The listing builds one solid part. Answer for the finished solid, in the listing's coordinates (mm). Give positions to 0.01 mm unless a question says otherwise; leave off trailing zeros. Write each loop counter-clockwise with the first axis right and the second up, starting at its lowest first coordinate (ties: lowest second). Pieces come first, ordered by that corner, then holes. Notation, with made-up numbers: (72, -26.5) - (101, -26.5) arc R33 ccw to (101, 12.5) - close; hole circle Ø4 at (63, -7). An arc over 180 degrees is marked (long way). Return JSON: item names as keys, results as strings.
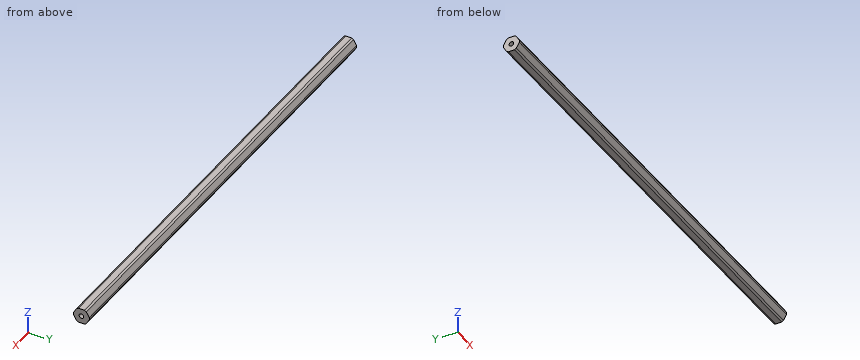
from build123d import *

# Parameters (mm, degrees)
BOSS_EXTRUDE1_DEPTH                  = 200.025
F_10_32_TAPPED_HOLE1_D               = 4.0386
F_10_32_TAPPED_HOLE1_DEPTH           = 16.34744
F_10_32_TAPPED_HOLE1_TIP             = 1.213317848
F_10_32_TAPPED_HOLE1_ON_FACE_2_D     = 4.0386
F_10_32_TAPPED_HOLE1_ON_FACE_2_DEPTH = 16.34744
F_10_32_TAPPED_HOLE1_ON_FACE_2_TIP   = 1.213317848


with BuildPart() as part:
    # Sketch1 → Boss-Extrude1 (new, symmetric)
    with BuildSketch(Plane(origin=(0, 0, 0), x_dir=(0, 0, -1), z_dir=(1, 0, 0))):
        with BuildLine():
            ThreePointArc((0.93173274, 6.79441227), (0, 6.858), (-0.93173274, 6.79441227))
            Line((-0.93173274, 6.79441227), (-5.41826726, 4.204110358))
            ThreePointArc((-5.41826726, 4.204110358), (-5.939202219, 3.429), (-6.35, 2.590301913))
            Line((-6.35, 2.590301913), (-6.35, -2.590301913))
            ThreePointArc((-6.35, -2.590301913), (-5.939202219, -3.429), (-5.41826726, -4.204110358))
            Line((-5.41826726, -4.204110358), (-0.93173274, -6.79441227))
            ThreePointArc((-0.93173274, -6.79441227), (0, -6.858), (0.93173274, -6.79441227))
            Line((0.93173274, -6.79441227), (5.41826726, -4.204110358))
            ThreePointArc((5.41826726, -4.204110358), (5.939202219, -3.429), (6.35, -2.590301913))
            Line((6.35, -2.590301913), (6.35, 2.590301913))
            ThreePointArc((6.35, 2.590301913), (5.939202219, 3.429), (5.41826726, 4.204110358))
            Line((5.41826726, 4.204110358), (0.93173274, 6.79441227))
        make_face()
    extrude(amount=BOSS_EXTRUDE1_DEPTH, both=True)

    # #10-32 Tapped Hole1
    with Locations(Plane(origin=(-200.025, 0, 0), x_dir=(0, 0, -1), z_dir=(-1, 0, 0))):
        with Locations((0, 0)):
            Hole(F_10_32_TAPPED_HOLE1_D / 2, depth=F_10_32_TAPPED_HOLE1_DEPTH)
            with Locations((0, 0, -(F_10_32_TAPPED_HOLE1_DEPTH + F_10_32_TAPPED_HOLE1_TIP / 2))):  # 118° drill point
                Cone(0, F_10_32_TAPPED_HOLE1_D / 2, F_10_32_TAPPED_HOLE1_TIP, mode=Mode.SUBTRACT)

    # #10-32 Tapped Hole1 on face 2
    with Locations(Plane(origin=(200.025, 0, 0), x_dir=(0, 0, 1), z_dir=(1, 0, 0))):
        with Locations((0, 0)):
            Hole(F_10_32_TAPPED_HOLE1_ON_FACE_2_D / 2, depth=F_10_32_TAPPED_HOLE1_ON_FACE_2_DEPTH)
            with Locations((0, 0, -(F_10_32_TAPPED_HOLE1_ON_FACE_2_DEPTH + F_10_32_TAPPED_HOLE1_ON_FACE_2_TIP / 2))):  # 118° drill point
                Cone(0, F_10_32_TAPPED_HOLE1_ON_FACE_2_D / 2, F_10_32_TAPPED_HOLE1_ON_FACE_2_TIP, mode=Mode.SUBTRACT)


solid = part.part
Item 1: A cutting plane is placed at A-A on x = 172.5. Determine the outline of the cut face in (y, z).
Answer below:
{"outline": "(-6.79, -0.93) - (-4.2, -5.42) arc R6.86 ccw to (-2.59, -6.35) - (2.59, -6.35) arc R6.86 ccw to (4.2, -5.42) - (6.79, -0.93) arc R6.86 ccw to (6.79, 0.93) - (4.2, 5.42) arc R6.86 ccw to (2.59, 6.35) - (-2.59, 6.35) arc R6.86 ccw to (-4.2, 5.42) - (-6.79, 0.93) arc R6.86 ccw to start"}
Item 2: Consider L1, parallel to Z at x = -184, y = 0.5; L2, parallel to Y at x = 191.75, z = 0; L3, parallel to Y at x = -91.5, z = -1.75. Determine where each line is inside the solid, lowest interval first.
Answer below:
{"L1": "z = -6.35 to -1.96, 1.96 to 6.35", "L2": "y = -6.86 to -2.02, 2.02 to 6.86", "L3": "y = -6.32 to 6.32"}
Item 3: Flat-ended cylindrical pins translate along their axes: P1, Ø2, axis at x = 52.5, y = -4, coming from the +Z side; P2, Ø1.5, axis at x = 90, z = -3, coming from the +Y side; P3, Ø2.5, axis at y = 0, z = 0, coming from the +X side. Find the tip coordinate at first contact, or state that the pin passes through.
Answer below:
{"P1": "stops at z = 6.17", "P2": "stops at y = 6.03", "P3": "stops at x = 183.22"}
